Source: CAD feature listing. Evaluate the final solid. Frame: model axes, mm. A direction names the side the tool comes from. Round coordinates to 2 decimals unless told otherwise and drop trailing zeros. Order: outer loops, then holes, each group sorted by start corner. A loop starts at its lowest first (then second) coordinate and runs counter-clockwise, first axis right, second up. Notation, with made-up numbers: (-29, 55) -> (1, 55) arc R26 ccw to (1, 90) -> close; hole circle Ø7 at (-23.5, 35). An arc over 180 degrees is marked (long way). Answer as CSV lines item,"result".
Autodesk Inventor part; units mm, degrees
ref_plane "YZ Plane" through (0, 0, 0) normal (1, 0, 0) x (0, 1, 0)
ref_plane "XZ Plane" through (0, 0, 0) normal (0, 1, 0) x (-1, 0, 0)
ref_plane "XY Plane" through (0, 0, 0) normal (0, 0, 1) x (1, 0, 0)
ref_plane "Work Plane1" through (0, 0, 0) normal (0, 0, 1) x (1, 0, 0)
sketch "Sketch1" plane through (0, 0, 0) normal (0, 0, 1) x (1, 0, 0)
  circle A0 centre (21.4625, 30.925) radius 2
  line L0 (0, 34.925) -> (25.4, 34.925)
  line L1 (0, 0) -> (0, 34.925)
  line L2 (0, 0) -> (2.54, 0)
  arc A1 (2.54, 0) -> (24.765, 0) centre (13.6525, 6.1484) ccw
  line L3 (24.765, 0) -> (24.765, 25.2044)
  arc A2 (24.765, 25.2044) -> (26.5659, 26.7312) centre (21.4625, 30.925) ccw
  spline S0 degree 3 poles (25.4, 34.925) (25.7861, 32.1988) (26.1753, 29.4627) (26.5659, 26.7312) knots -1.120112 -1.120112 -1.120112 -1.120112 -0.293842 -0.293842 -0.293842 -0.293842
  circle A3 centre (4, 30.925) radius 2
  circle A4 centre (21.4625, 30.925) radius 2
  circle A5 centre (21.4625, 30.925) radius 4
  circle A6 centre (4, 30.925) radius 2
  circle A7 centre (4, 30.925) radius 4
  line L4 (21.4625, 34.925) -> (4, 34.925)
  line L5 (4, 34.925) -> (4, 26.925)
  line L6 (4, 26.925) -> (21.4625, 26.925)
  line L7 (21.4625, 26.925) -> (21.4625, 34.925)
  line L8 (-4.0963, 34.925) -> (-4.0963, 26.925)
  line L9 (4, 34.925) -> (-4.0963, 34.925)
  line L10 (4, 26.925) -> (-4.0963, 26.925)
  line L11 (-4.0963, 34.925) -> (-0.9213, 34.925)
  line L12 (-0.9213, 34.925) -> (-0.9213, 26.925)
  line L13 (-0.9213, 26.925) -> (-4.0963, 26.925)
  line L14 (-4.0963, 26.925) -> (-4.0963, 34.925)
  circle A8 centre (12.7313, 10.2875) radius 7.9375
  point P0 (-20.6063, 34.925)
  dimension "d0" = 16.51
  dimension "d1" = 3.175
  dimension "d2" = 8
extrude "Extrusion1" add sketch "Sketch1" along normal blind 3.175 contours A0 L7 | A0 L7 A5 | L7 A0 | A0 L7 A5 | A5 L6 A7 L0 | A7 L1 L0 | L5 A3 A7 | A7 L5 A3 | L10 L1 A7 | L1 L10 L12 L9 | L5 A3 | A3 L5 | L12 L10 L8 L9
sketch "Sketch2" plane through (0, 0, 3.175) normal (0, 0, 1) x (1, 0, 0)
  line L0 (-0.9213, 34.925) -> (-0.9213, 26.925)
  line L1 (-4.0963, 34.925) -> (-4.0963, 26.925)
  line L2 (4, 26.925) -> (-4.0963, 26.925)
  line L3 (4, 34.925) -> (-4.0963, 34.925)
  point P0 (0, 0)
extrude "Extrusion2" add sketch "Sketch2" along normal blind 12.7
fillet "Fillet1" radius 3.9878 2 edges at (-2.5088, 34.925, 15.875) (-2.5088, 26.925, 15.875)
sketch "Sketch3" plane through (-0.9213, 26.925, 3.175) normal (1, 0, 0) x (0, 0, -1)
  line L0 (0, 8) -> (0, 0)
  point P0 (3.175, -26.925)
  point P1 (-6.35, 4)
  point P2 (0, 4)
  point P3 (0, 4)
  dimension "d8" = 6.35
hole "Hole1" at (-0.9213, 30.925, 9.525) direction (-1, 0, 0) diameter 4 end through all
sketch "Sketch6" plane through (0, 0, 3.175) normal (0, 0, 1) x (1, 0, 0)
  circle A0 centre (21.4625, 30.925) radius 2
  line L0 (0, 34.925) -> (25.4, 34.925)
  line L1 (0, 0) -> (0, 34.925)
  line L2 (0, 0) -> (2.54, 0)
  arc A1 (2.54, 0) -> (24.765, 0) centre (13.6525, 6.1484) ccw
  line L3 (24.765, 0) -> (24.765, 25.2044)
  arc A2 (24.765, 25.2044) -> (26.5659, 26.7312) centre (21.4625, 30.925) ccw
  spline S0 degree 3 poles (25.4, 34.925) (25.7861, 32.1988) (26.1753, 29.4627) (26.5659, 26.7312) knots -1.120112 -1.120112 -1.120112 -1.120112 -0.293842 -0.293842 -0.293842 -0.293842
  circle A3 centre (4, 30.925) radius 2
  circle A4 centre (12.7313, 10.2875) radius 7.9375
  point P0 (21.4625, 30.925)
  point P1 (4, 30.925)
hole "Hole2" at (21.4625, 30.925, 3.175) at (4, 30.925, 3.175) direction (0, 0, -1) diameter 4 end through all both
chamfer "Chamfer5" distance 1.5875 angle 45 1 edges at (-0.9213, 30.925, 3.175)
chamfer "Chamfer6" distance 1.5875 angle 45 1 edges at (-4.0963, 30.925, 0)
sketch "Sketch7" plane through (-4.0963, 26.925, 1.5875) normal (-1, 0, 0) x (0, 0, 1)
  circle A0 centre (7.9375, 4) radius 2
  circle A1 centre (7.9375, 4) radius 4
  line L0 (3.175, 8) -> (10.2997, 8)
  point P0 (-1.5875, -26.925)
extrude "Extrusion5" add sketch "Sketch7" along normal blind 0.5
properties part number "Sensor Mount"
1. Reachability of faces 1 (the flat face through (-4.596, 29, 11)), 2 (the flat face through (13, 31, 3.175)), 3 (the flat face through (-4.096, 31, 14)) from +Z, -Z, +X, -X, +Y, -Y: full face, straight path, thin tool, end or side. Return the list, or none.
Results below:
face 1,"+Z, -Z, -X, +Y, -Y"
face 2,"+Z, +X, +Y, -Y"
face 3,"+Z, -X"
2. Mould query, pull axis Y, two halves, no side actions, for faces 4 (the cylindrical face through (-2.531, 33.726, 14.738)), 5 (the cylindrical face through (-4.34, 29.72, 13.34)), 6 (the cylindrical face through (22, 29, 2)), 7 (the flat face through (11, 31, 0)). Classes: released by +Y, released by -Y, zero draft, split by the parting line, or undercut.
Results below:
face 4,"released by +Y"
face 5,"split by the parting line"
face 6,"undercut"
face 7,"zero draft"
3. Section query A-A on x = 4. Return loops of the section in (y, z) (3 decimals).
Results below:
outline,"(26.925, 0) -> (28.925, 0) -> (28.925, 3.175) -> (26.925, 3.175) -> close; (32.925, 0) -> (34.925, 0) -> (34.925, 3.175) -> (32.925, 3.175) -> close"
4. Pin query (flat end, axial travel): pin 1 (4.5 mm diameter, centred on y = 30.925, z = 9.525, fed in from +X). Return the tip coordinate at first contact, or that it passes through.
Results below:
pin 1,"x = -0.92"
5. Section query B-B on y = 30.25. Return loops of the section in (x, z) (1 decimal).
Results below:
outline,"(-4.6, 5.6) -> (-4.1, 5.6) -> (-4.1, 1.6) -> (-2.5, 0) -> (2.1, 0) -> (2.1, 3.2) -> (0.7, 3.2) -> (-0.9, 4.8) -> (-0.9, 7.6) -> (-4.6, 7.6) -> close; (-4.6, 11.4) -> (-0.9, 11.4) -> (-0.9, 15.8) -> (-4.1, 15.8) -> (-4.1, 13.5) -> (-4.6, 13.5) -> close; (5.9, 0) -> (19.6, 0) -> (19.6, 3.2) -> (5.9, 3.2) -> close; (23.3, 0) -> (25.4, 0) -> (25.4, 3.2) -> (23.3, 3.2) -> close"
6. Line query: L1, parallel to Y at x = 4, z = 0.7 (3 decimals); L2, parallel to X at y = 30, z = 7.25; L3, parallel to Z at x = 24, y = 29.25 (3 decimals). Output: solid intervals per line, ascending. Write a range as [from, to].
Results below:
L1,"[26.925, 28.925], [32.925, 34.925]"
L2,"[-4.6, -0.92]"
L3,"[0, 3.175]"
7. Section query D-D on y = 33.25. Return loops of the section in (x, z) (1 decimal), and give its area (3 significant figures).
Results below:
outline,"(-4.6, 6.3) -> (-4.1, 6.3) -> (-4.1, 1.6) -> (-2.5, 0) -> (24.7, 0) -> (24.7, 3.2) -> (0.7, 3.2) -> (-0.9, 4.8) -> (-0.9, 15.1) -> (-4.1, 15.1) -> (-4.1, 12.8) -> (-4.6, 12.8) -> close"
area,"133 mm2"
8. Section query C-C on z = 8.25. Return loops of the section in (x, y) (3 decimals), and give its area (3 significant figures).
Results below:
outline,"(-4.596, 27.134) -> (-4.096, 27.134) -> (-4.096, 26.925) -> (-0.921, 26.925) -> (-0.921, 29.384) -> (-4.596, 29.384) -> close; (-4.596, 32.466) -> (-0.921, 32.466) -> (-0.921, 34.925) -> (-4.096, 34.925) -> (-4.096, 34.716) -> (-4.596, 34.716) -> close"
area,"17.9 mm2"
